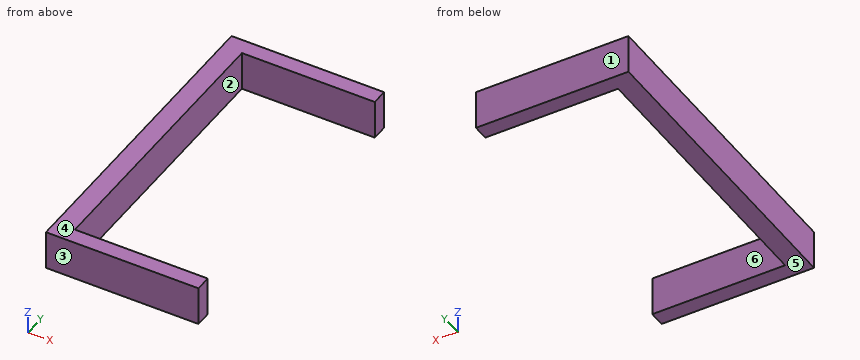
from build123d import *

# Parameters (mm, degrees)
F5_W     = 101.6
F5_H     = 12.7
F6_DEPTH = 6.35
F7_W     = 5.08
F7_H     = 12.7
F8_DEPTH = 42.926


# Not quite as in the source:
# - a feature of the source that left no trace in its solid (it failed there, or was rolled back) is left out


with BuildPart() as f6:
    # F5 (on Right) → F6 (new body)
    with BuildSketch(Plane.YZ):
        with Locations((-2.5232887447, 14.3209207639)):
            Rectangle(F5_W, F5_H)
    extrude(amount=F6_DEPTH)

    # F7 (on face) → F8 (join)
    with BuildSketch(Plane.YZ.offset(6.35)):
        with Locations((-50.7832887447, 14.3209207639)):
            Rectangle(F7_W, F7_H)
        with Locations((45.7367112553, 14.3209207639)):
            Rectangle(F7_W, F7_H)
    extrude(amount=F8_DEPTH)


solid = f6.part
For this review, take the finished solid that the model builds, in its own axes (mm). Face numbers are marked on the shaded views. A direction names the side the tool comes from. Give positions to 0.01 mm unless a question says otherwise; leave off trailing zeros. Loops run counter-clockwise (first coordinate to the right, second up) from the corner with the lowest first, then second, coordinate; pieces in that order, holes last. Notation, with made-up numbers: (-32, 8.25) -> (-17, 8.25) arc R31 cw to (-17, 44.25) -> close; hole circle Ø2 at (83.5, 46.5). An arc over 180 degrees is marked (long way). One line per question, with ' | ' between items.
1) We need section B-B (z = 19.25). Write out the cut boundary in (x, y).
Resolved:
outline: (0, -53.32) -> (49.28, -53.32) -> (49.28, -48.24) -> (6.35, -48.24) -> (6.35, 43.2) -> (49.28, 43.2) -> (49.28, 48.28) -> (0, 48.28) -> close
2) To check wall thickness, follow probe 1 along Y at (x, z) = (32.5, 16); probe 2 along X at (y, z) = (-40, 19). State the ranges of each line that lie inside material, in increasing order.
Resolved:
probe 1: y = -53.32 to -48.24, 43.2 to 48.28 | probe 2: x = 0 to 6.35
3) We need section A-A (x = 21). Write out the cut boundary in (y, z), plus the area to 3 significant figures.
Resolved:
outline: (-53.32, 7.97) -> (-48.24, 7.97) -> (-48.24, 20.67) -> (-53.32, 20.67) -> close; (43.2, 7.97) -> (48.28, 7.97) -> (48.28, 20.67) -> (43.2, 20.67) -> close | area: 129 mm2
4) Insertion check: pin 1 Ø4 at (y, z) = (0, 16) entering from +X. The pin has a flat end and moves straight along its axis. Give the tip position at first contact, or say it passes through.
Resolved:
pin 1: stops at x = 6.35
5) For the marked faces 5 and 6, list the 3-axis set-ups (+Z, -Z, +X, -X, +Y, -Y) from which the entire face can be reached by the end or side of a thin tool; tool diameter is ignored.
Resolved:
face 5: -Z, +X, -X, +Y, -Y | face 6: +Z, -Z, +X
6) We need section C-C (y = 1). Write out the cut boundary in (x, z), plus the area to 3 significant figures.
Resolved:
outline: (0, 7.97) -> (6.35, 7.97) -> (6.35, 20.67) -> (0, 20.67) -> close | area: 80.6 mm2
7) The part is to be moulded in two halves that separate along Y. For the marked faces 1, 2, 3 and 4, say which applies: +Y half, -Y half, draft (parallel to the pull), parting line (faces both ways), or undercut.
Resolved:
face 1: +Y half | face 2: undercut | face 3: -Y half | face 4: draft
